CAD build for the part. Positions are in the model's coordinates, mm. A direction names the side the tool comes from. Coordinates: 2 decimals unless noted, no trailing zeros. Order: outer loops, then holes, each group sorted by start corner. A loop starts at its lowest first (then second) coordinate and runs counter-clockwise, first axis right, second up. Notation, with made-up numbers: (4, 4.5) - (24, 4.5) arc R8 cw to (24, 12.5) - close; hole circle Ø4 at (37, -9.5). An arc over 180 degrees is marked (long way). Use one line per item in the form item = value.
```python
from build123d import *

# Parameters (mm, degrees)
F1_DEPTH = 7.62
F2_DEPTH = 3.81


with BuildPart() as f1:
    # F0 (on Front) → F1 (new body)
    with BuildSketch(Plane.XZ):
        Polygon((-20.32, 13.97), (-20.32, -19.05), (-10.16, -19.05), (-10.16, 3.81), (10.16, 3.81), (10.16, -19.05), (20.32, -19.05), (20.32, 13.97), align=None)
    extrude(amount=F1_DEPTH)

    # F0 (on Front) → F2 (join)
    with BuildSketch(Plane.XZ):
        Polygon((25.4, 19.05), (-25.4, 19.05), (-25.4, -19.05), (-20.32, -19.05), (-20.32, 13.97), (20.32, 13.97), (20.32, -19.05), (25.4, -19.05), align=None)
        Polygon((-10.16, 3.81), (-10.16, -19.05), (-5.08, -19.05), (-5.08, -1.27), (5.08, -1.27), (5.08, -19.05), (10.16, -19.05), (10.16, 3.81), align=None)
        Polygon((-20.32, -19.05), (-25.4, -19.05), (-25.4, -24.13), (-5.08, -24.13), (-5.08, -19.05), (-10.16, -19.05), align=None)
        Polygon((25.4, -24.13), (25.4, -19.05), (20.32, -19.05), (10.16, -19.05), (5.08, -19.05), (5.08, -24.13), align=None)
    extrude(amount=F2_DEPTH)


solid = f1.part
```
Item 1: Drop flat-ended pins along their axis: pin 1 (1.1 mm diameter, centred on x = -1, y = -5.5, fed in from +Z); pin 2 (5 mm diameter, centred on x = 14, z = -9, fed in from +Y); pin 3 (1.9 mm diameter, centred on y = -5.5, z = -2, fed in from -X); pin 4 (1.1 mm diameter, centred on x = 1, y = -1.5, fed in from -Z). Give the stop position or say it passes through.
Derived:
pin_1 = 13.97
pin_2 = 0
pin_3 = -20.32
pin_4 = -1.27
Item 2: Cut at C-C, the plane y = -1.5. Write the cut outline in (x, z).
Derived:
outline = (-25.4, -24.13) - (-5.08, -24.13) - (-5.08, -1.27) - (5.08, -1.27) - (5.08, -24.13) - (25.4, -24.13) - (25.4, 19.05) - (-25.4, 19.05) - close
Item 3: Cut at B-B, the plane x = -18.5. Write the cut outline in (y, z), plus the area to 3 significant figures.
Derived:
outline = (-7.62, -19.05) - (-3.81, -19.05) - (-3.81, -24.13) - (0, -24.13) - (0, 19.05) - (-3.81, 19.05) - (-3.81, 13.97) - (-7.62, 13.97) - close
area = 290 mm²
Item 4: Cut at D-D, the plane z = 15. Write the cut outline in (x, y), plus the area to 3 significant figures.
Derived:
outline = (-25.4, -3.81) - (25.4, -3.81) - (25.4, 0) - (-25.4, 0) - close
area = 194 mm²
Item 5: Cut at A-A, the plane z = -11.5. Write the cut outline in (x, y), plus the area to 3 significant figures.
Derived:
outline = (-25.4, -3.81) - (-20.32, -3.81) - (-20.32, -7.62) - (-10.16, -7.62) - (-10.16, -3.81) - (-5.08, -3.81) - (-5.08, 0) - (-25.4, 0) - close; (5.08, -3.81) - (10.16, -3.81) - (10.16, -7.62) - (20.32, -7.62) - (20.32, -3.81) - (25.4, -3.81) - (25.4, 0) - (5.08, 0) - close
area = 232 mm²
Item 6: Drill centre lines: line 1 (X direction, y = -3.75, z = -20.5); line 2 (X direction, y = -5.5, z = -13); line 3 (X direction, y = -6.75, z = 9.5). Where is each one in solid material? Low to high. Write a range as [from, to].
Derived:
line_1 = [-25.4, -5.08], [5.08, 25.4]
line_2 = [-20.32, -10.16], [10.16, 20.32]
line_3 = [-20.32, 20.32]
Item 7: Two-plate mould, pull along X, no slides. Class faces 1 (the face through (-5.08, -2, -13)), 2 (the face through (-15, -2, -24.13)), 3 (the face through (25.4, -2, -3)): +X half, -X half, draft (parallel to the pull), parting line (faces both ways), or undercut.
Derived:
face_1 = undercut
face_2 = draft
face_3 = +X half
Item 8: 3-axis set-ups, long thin cutter, end or side, ignore diameter. For faces 4 (the face through (-20.32, -6, -2)), 5 (the face through (15, -6, -19.05)), 6 (the face through (0, -6, 13.97)), 7 (the face through (-10.16, -6, -8)), 8 (the face through (0, -2, -1.27)): which of +Z, -Z, +X, -X, +Y, -Y reach the whole face in a straight line?
Derived:
face_4 = +Z, -Z, -X, -Y
face_5 = -Z, +X, -X, -Y
face_6 = +Z, +X, -X, -Y
face_7 = -Z, -Y
face_8 = -Z, +Y, -Y
